Input: part model. Units: mm. Frame: model coordinates. Coordinates: 2 decimals unless noted, no trailing zeros. Write each loop counter-clockwise with the first axis right and the second up, starting at its lowest first coordinate (ties: lowest second). Pieces come first, ordered by that corner, then holes. Notation, with made-up numbers: M 83,-17.75 L 104,-17.75 A26 ccw 104,10.25 Z; hole C 62,30.25 d5. An arc over 180 degrees is marked long. Use one line per item in the form item = value.
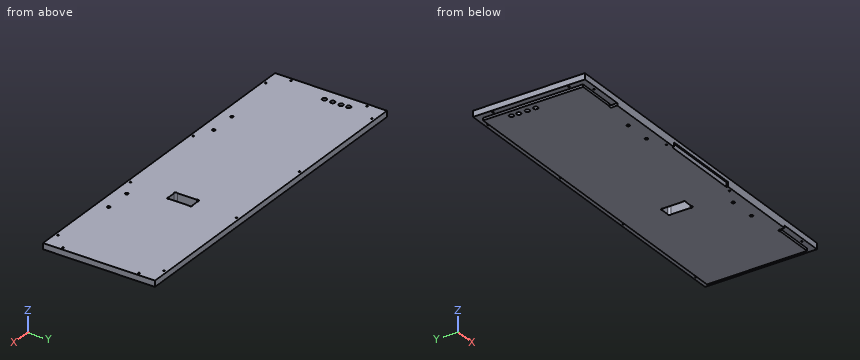
from build123d import *

# Parameters (mm, degrees)
BACKOUTLINE_W               = 728.6625
BACKOUTLINE_H               = 238.125
BACKOUTLINE_THICKNESS_DEPTH = 17.78
BCAKHOLES_R                 = 1.5875
BCAKHOLES_R_2               = 3.175
BCAKHOLES_W                 = 25.4
BCAKHOLES_H                 = 50.8
CUT_EXTRUDE1_DEPTH          = 17.78
SKETCH6_R                   = 3.302
CUT_EXTRUDE4_DEPTH          = 17.78
BACKPOWERBOXLIP_W           = 169.8625
BACKPOWERBOXLIP_H           = 9.525
CUT_EXTRUDE2_DEPTH          = 3.175
CUT_EXTRUDE3_DEPTH          = 5.08
SKETCH7_R                   = 3.302
CUT_EXTRUDE5_DEPTH          = 5.08
BACKAMPACCESSHOLES_R        = 4.7625
CUT_EXTRUDE6_DEPTH          = 17.78


with BuildPart() as part:
    # BackOutline → BackOutline_Thickness (new body)
    with BuildSketch(Plane.XY):
        with Locations((-5376.06875, 779.4625)):
            Rectangle(BACKOUTLINE_W, BACKOUTLINE_H)
    extrude(amount=-BACKOUTLINE_THICKNESS_DEPTH)

    # BcakHoles → Cut-Extrude1 (cut)
    with BuildSketch(Plane.XY):
        with Locations((-5702.3, 892.175)):
            Circle(BCAKHOLES_R)
        with Locations((-5734.05, 860.425)):
            Circle(BCAKHOLES_R)
        with Locations((-5734.05, 698.5)):
            Circle(BCAKHOLES_R)
        with Locations((-5702.3, 666.75)):
            Circle(BCAKHOLES_R)
        with Locations((-5569.74375, 684.2125)):
            Circle(BCAKHOLES_R_2)
        with Locations((-5512.59375, 684.2125)):
            Circle(BCAKHOLES_R_2)
        with Locations((-5474.890625, 666.75)):
            Circle(BCAKHOLES_R)
        with Locations((-5277.246875, 666.75)):
            Circle(BCAKHOLES_R)
        with Locations((-5239.54375, 684.2125)):
            Circle(BCAKHOLES_R_2)
        with Locations((-5182.39375, 684.2125)):
            Circle(BCAKHOLES_R_2)
        with Locations((-5049.8375, 666.75)):
            Circle(BCAKHOLES_R)
        with Locations((-5018.0875, 698.5)):
            Circle(BCAKHOLES_R)
        with Locations((-5018.0875, 860.425)):
            Circle(BCAKHOLES_R)
        with Locations((-5049.8375, 892.175)):
            Circle(BCAKHOLES_R)
        with Locations((-5277.246875, 892.175)):
            Circle(BCAKHOLES_R)
        with Locations((-5474.890625, 892.175)):
            Circle(BCAKHOLES_R)
        with Locations((-5278.4375, 777.875)):
            Rectangle(BCAKHOLES_W, BCAKHOLES_H)
    extrude(amount=-CUT_EXTRUDE1_DEPTH, mode=Mode.SUBTRACT)

    # Sketch6 → Cut-Extrude4 (cut)
    with BuildSketch(Plane.XY):
        with Locations((-5288.802633409, 800.940133409)):
            Circle(SKETCH6_R)
        with Locations((-5268.072366591, 800.940133409)):
            Circle(SKETCH6_R)
        with Locations((-5288.802633409, 754.809866591)):
            Circle(SKETCH6_R)
        with Locations((-5268.072366591, 754.809866591)):
            Circle(SKETCH6_R)
    extrude(amount=-CUT_EXTRUDE4_DEPTH, mode=Mode.SUBTRACT)

    # BackPowerBoxLip → Cut-Extrude2 (cut)
    with BuildSketch(Plane.XZ.offset(-660.4)):
        with Locations((-5376.06875, -13.0175)):
            Rectangle(BACKPOWERBOXLIP_W, BACKPOWERBOXLIP_H)
    extrude(amount=-CUT_EXTRUDE2_DEPTH, mode=Mode.SUBTRACT)

    # BackLedge → Cut-Extrude3 (cut)
    with BuildSketch(Plane(origin=(0, 0, -17.78), x_dir=(-1, 0, 0), z_dir=(0, 0, -1))):
        Polygon((5011.7375, 660.4), (5113.3375, 660.4), (5113.3375, 673.1), (5024.4375, 673.1), (5024.4375, 885.825), (5727.7, 885.825), (5727.7, 673.1), (5638.8, 673.1), (5638.8, 660.4), (5740.4, 660.4), (5740.4, 898.525), (5011.7375, 898.525), align=None)
    extrude(amount=-CUT_EXTRUDE3_DEPTH, mode=Mode.SUBTRACT)

    # Sketch7 → Cut-Extrude5 (cut)
    with BuildSketch(Plane(origin=(0, 0, -17.78), x_dir=(-1, 0, 0), z_dir=(0, 0, -1))):
        with Locations((5641.525003649, 671.235178531)):
            Circle(SKETCH7_R)
        with Locations((5110.612496351, 671.235178531)):
            Circle(SKETCH7_R)
    extrude(amount=-CUT_EXTRUDE5_DEPTH, mode=Mode.SUBTRACT)

    # BackAmpAccessHoles → Cut-Extrude6 (cut)
    with BuildSketch(Plane(origin=(0, 0, -17.78), x_dir=(-1, 0, 0), z_dir=(0, 0, -1))):
        with Locations((5713.73, 835.025)):
            Circle(BACKAMPACCESSHOLES_R)
        with Locations((5712.46, 819.785)):
            Circle(BACKAMPACCESSHOLES_R)
        with Locations((5712.46, 802.005)):
            Circle(BACKAMPACCESSHOLES_R)
        with Locations((5712.46, 784.225)):
            Circle(BACKAMPACCESSHOLES_R)
    extrude(amount=-CUT_EXTRUDE6_DEPTH, mode=Mode.SUBTRACT)


solid = part.part
(1) Section query A-A on x = -5361.5. Return the cut outline in (y, z) (3 decimals).
Computed:
outline = M 660.4,-8.255 L 663.575,-8.255 L 663.575,-17.78 L 885.825,-17.78 L 885.825,-12.7 L 898.525,-12.7 L 898.525,0 L 660.4,0 Z
(2) Section query B-B on x = -5101. Return the cut outline in (y, z) (3 decimals).
Computed:
outline = M 660.4,-12.7 L 673.1,-12.7 L 673.1,-17.78 L 885.825,-17.78 L 885.825,-12.7 L 898.525,-12.7 L 898.525,0 L 660.4,0 Z
(3) First-contact query: pin 1 Ø4 at (y, z) = (664, -15.5) entering from +X; pin 2 Ø3.5 at (x, y) = (-5734.05, 698.5) entering from -Z; pin 3 Ø5 at (x, z) = (-5346, -14) entering from -Y (3 decimals). Flat tips, straight axial feed; report the tip coordinate or a pass-through.
Computed:
pin_1 = -5113.34
pin_2 = -12.7
pin_3 = 663.575
(4) Line query: probe 1 along X at (y, z) = (784, -11.75); probe 2 along Y at (x, z) = (-5284.5, -4.75) (3 decimals); probe 3 along X at (y, z) = (767, -3.25). Output: solid intervals per line, ascending.
Computed:
probe_1 = -5740.4 to -5717.22, -5707.7 to -5291.14, -5265.74 to -5011.74
probe_2 = 660.4 to 752.475, 803.275 to 898.525
probe_3 = -5740.4 to -5291.14, -5265.74 to -5011.74
(5) Section query C-C on x = -5586. Return the cut outline in (y, z) (3 decimals).
Computed:
outline = M 660.4,-17.78 L 885.825,-17.78 L 885.825,-12.7 L 898.525,-12.7 L 898.525,0 L 660.4,0 Z
